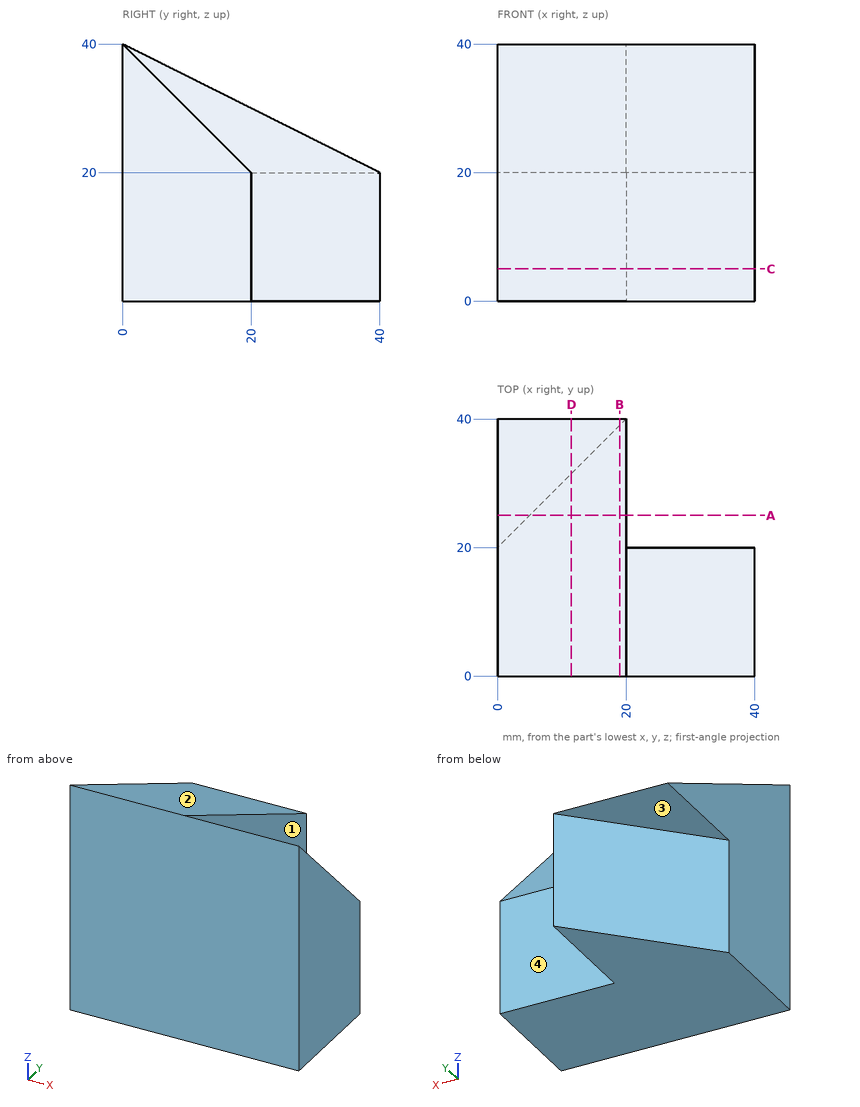
Here's the drawing with two shaded views (mm, measured from the low corner). I have some questions. A direction names the side the tool comes from. Give positions to 0.01 mm unless a question says otherwise; leave off trailing zeros. Order: outer loops, then holes, each group sorted by start corner. A loop starts at its lowest first (then second) coordinate and runs counter-clockwise, first axis right, second up. Notation, with made-up numbers: (47, 53) - (79, 53) arc R37 cw to (79, 90) - close; hole circle Ø2 at (66, 84.25). An arc over 180 degrees is marked (long way). Use a Markdown table: item, result. Add a question column.
Q1. If we section it at C-C on z = 5: Write out the boundary of the cut face in (x, y).
Q2. If we section it at B-B on x = 19: Write out the boundary of the cut face in (y, z), plus the area to 3 significant figures.
Q3. I'm going to push flat-ended pins straight in: pin 1 (6 mm diameter, centred on x = 5, y = 31.5, fed in from -Z); pin 2 (3 mm diameter, centred on y = 33.5, z = 13, fed in from -X); pin 3 (6 mm diameter, centred on x = 31, z = 6.5, fed in from +Y). Where does each tip first touch, or does it pass through?
Q4. If we section it at A-A on y = 25: Write out the boundary of the cut face in (x, z), plus the area to 3 significant figures.
Q5. Please list where these lines run through material, in increasing order: line 1 along Y through (x, z) = (23.5, 8); line 2 along Y through (x, z) = (26.5, 27).
Q6. On a 3-axis mill with a long thin cutter (end or side, diameter ignored), from which of +Z, -Z, +X, -X, +Y, -Y can I reach the whole of each face in a straight line? I mean the marked faces 1, 2, 3 and 4. Say none if no direction works.
Q7. If we section it at D-D on x = 11.5: Write out the boundary of the cut face in (y, z).
Answers follow:
| question | item | result |
|---|---|---|
| 1 | outline | (0, 0) - (40, 0) - (40, 20) - (20, 20) - (20, 40) - (0, 20) - close |
| 2 | outline | (0, 0) - (39, 0) - (39, 20) - (40, 20) - (0, 40) - close |
| 2 | area | 1,180 mm^2 |
| 3 | pin 1 | stops at z = 20 |
| 3 | pin 2 | stops at x = 12 |
| 3 | pin 3 | stops at y = 20 |
| 4 | outline | (0, 20) - (5, 20) - (5, 0) - (20, 0) - (20, 27.5) - (0, 27.5) - close |
| 4 | area | 450 mm^2 |
| 5 | line 1 | y = 0 to 20 |
| 5 | line 2 | y = 0 to 13 |
| 6 | face 1 | +Z, +X, +Y |
| 6 | face 2 | +Z, +X, -X, +Y |
| 6 | face 3 | -Z, -X, +Y |
| 6 | face 4 | +Z, -Z, +X, +Y |
| 7 | outline | (0, 0) - (31.5, 0) - (31.5, 20) - (40, 20) - (0, 40) - close |
